For this review, use the dimensioned drawing (mm, ordinates from the lowest corner) and the shaded views. Coordinates: 2 decimals unless noted, no trailing zeros. Loops run counter-clockwise (first coordinate to the right, second up) from the corner with the lowest first, then second, coordinate; pieces in that order, holes last. Notation, with made-up numbers: (-14.75, 62.5) - (35.25, 62.5) arc R31 cw to (35.25, 91.5) - close; hole circle Ø5 at (39.25, 68.5). An arc over 180 degrees is marked (long way). Return JSON: item names as keys, results as strings. Group by question number.
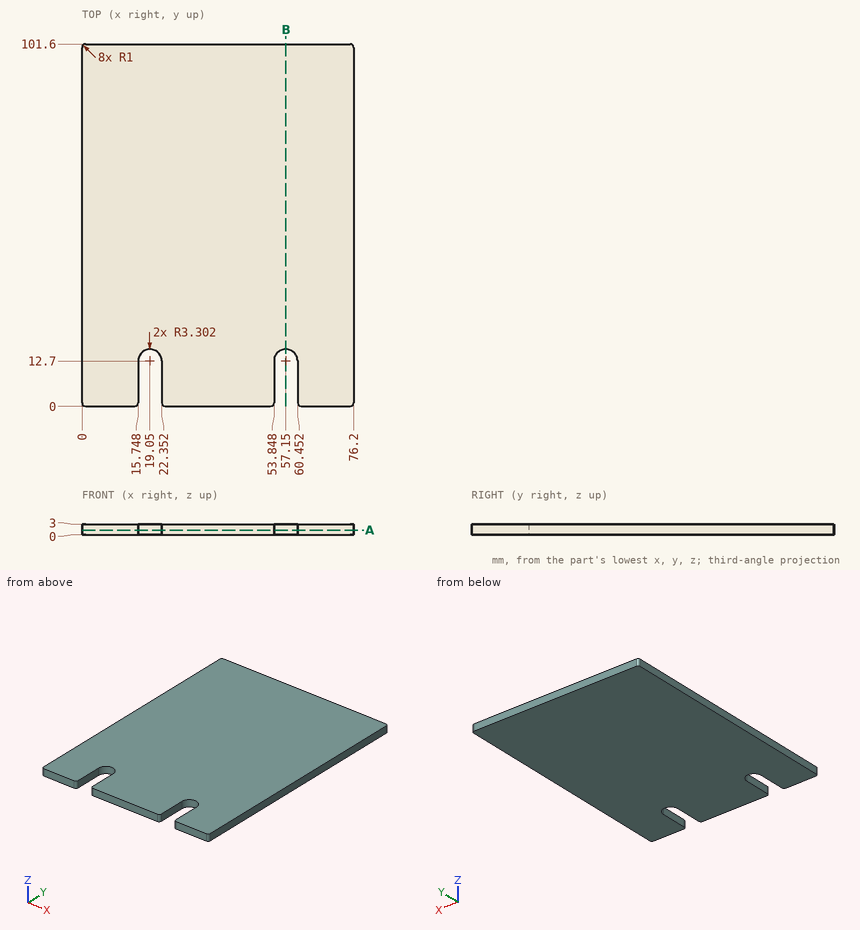
Item 1: Add section A-A (z = 1.35). State the section outline as (x, y) points, then the cut area to 3 significant figures.
Item 2: Add section B-B (x = 57.15). State the section outline as (y, z) points.
Item 3: To check wall thickness, follow line 1 (X direction, y = 8, z = 0.45); line 2 (Y direction, x = 57, z = 1.6); line 3 (Y direction, x = 15, z = 2.2). State the ranges of each line that lie inside material, in increasing order. Write a range as from..to.
Answers below:
{
 "1": {"outline": "(0, 1) arc R1 ccw to (1, 0) - (14.75, 0) arc R1 ccw to (15.75, 1) - (15.75, 12.7) arc R3.3 cw to (22.35, 12.7) - (22.35, 1) arc R1 ccw to (23.35, 0) - (52.85, 0) arc R1 ccw to (53.85, 1) - (53.85, 12.7) arc R3.3 cw to (60.45, 12.7) - (60.45, 1) arc R1 ccw to (61.45, 0) - (75.2, 0) arc R1 ccw to (76.2, 1) - (76.2, 100.6) arc R1 ccw to (75.2, 101.6) - (1, 101.6) arc R1 ccw to (0, 100.6) - close", "area": "7,540 mm^2"},
 "2": {"outline": "(16, 0) - (101.6, 0) - (101.6, 3) - (16, 3) - close"},
 "3": {"line 1": "x = 0..15.75, 22.35..53.85, 60.45..76.2", "line 2": "y = 16..101.6", "line 3": "y = 0.03..101.6"}
}
